Autodesk Inventor part; units mm, degrees
ref_plane "YZ Plane" through (0, 0, 0) normal (1, 0, 0) x (0, 1, 0)
ref_plane "XZ Plane" through (0, 0, 0) normal (0, 1, 0) x (-1, 0, 0)
ref_plane "XY Plane" through (0, 0, 0) normal (0, 0, 1) x (1, 0, 0)
sketch "Szkic1" plane through (0, 0, 0) normal (0, 0, 1) x (1, 0, 0)
  line L0 (-218.2, 284.6) -> (218.2, 284.6)
  line L1 (219.2, 283.6) -> (219.2, 0.3)
  line L2 (218.2, -0.7) -> (-218.2, -0.7)
  line L3 (-219.2, 0.3) -> (-219.2, 283.6)
  arc A0 (219.2, 283.6) -> (218.2, 284.6) centre (218.2, 283.6) ccw
  arc A1 (-218.2, 284.6) -> (-219.2, 283.6) centre (-218.2, 283.6) ccw
  arc A2 (-219.2, 0.3) -> (-218.2, -0.7) centre (-218.2, 0.3) ccw
  arc A3 (218.2, -0.7) -> (219.2, 0.3) centre (218.2, 0.3) ccw
  line L4 (214.5, 280.9) -> (-214.5, 280.9)
  line L5 (-215.5, 279.9) -> (-215.5, 3.3625)
  line L6 (-214.5, 2.3625) -> (214.5, 2.3625)
  line L7 (215.5, 3.3625) -> (215.5, 279.9)
  arc A4 (-214.5, 280.9) -> (-215.5, 279.9) centre (-214.5, 279.9) ccw
  arc A5 (215.5, 279.9) -> (214.5, 280.9) centre (214.5, 279.9) ccw
  arc A6 (214.5, 2.3625) -> (215.5, 3.3625) centre (214.5, 3.3625) ccw
  arc A7 (-215.5, 3.3625) -> (-214.5, 2.3625) centre (-214.5, 3.3625) ccw
  point P0 (0, 0)
  point P1 (219.2, 284.6)
  point P2 (-219.2, -0.7)
  point P3 (219.2, -0.7)
  dimension "d7" = 1
extrude "Wyciągnięcie proste1" add sketch "Szkic1" along normal blind 1.5
sketch "Szkic2" plane through (0, 0, 0) normal (0, 0, -1) x (-1, 0, 0)
  line L0 (217, 2.5) -> (217, 281.4)
  line L1 (216, 282.4) -> (-216, 282.4)
  line L2 (-217, 281.4) -> (-217, 2.5)
  line L3 (-215.5, 3.3625) -> (-215.5, 279.9)
  arc A0 (-214.5, 280.9) -> (-215.5, 279.9) centre (-214.5, 279.9) ccw
  line L4 (-214.5, 280.9) -> (214.5, 280.9)
  arc A1 (215.5, 279.9) -> (214.5, 280.9) centre (214.5, 279.9) ccw
  line L5 (215.5, 279.9) -> (215.5, 3.3625)
  arc A2 (214.5, 2.3625) -> (215.5, 3.3625) centre (214.5, 3.3625) ccw
  line L6 (216, 1.5) -> (73, 1.5)
  line L7 (214.5, 2.3625) -> (-214.5, 2.3625)
  arc A3 (-215.5, 3.3625) -> (-214.5, 2.3625) centre (-214.5, 3.3625) ccw
  line L8 (-51.8, 1.5) -> (-216, 1.5)
  line L9 (-216, 282.4) -> (-215.9969, 282.4)
  line L10 (-39.9, 1.5) -> (-51.8, 1.5)
  line L11 (61.1, 1.5) -> (-39.9, 1.5)
  line L12 (73, 1.5) -> (61.1, 1.5)
  arc A4 (-216, 282.4) -> (-217, 281.4) centre (-216, 281.4) ccw
  arc A5 (217, 281.4) -> (216, 282.4) centre (216, 281.4) ccw
  arc A6 (216, 1.5) -> (217, 2.5) centre (216, 2.5) ccw
  arc A7 (-217, 2.5) -> (-216, 1.5) centre (-216, 2.5) ccw
  point P0 (0, 0)
  dimension "d10" = 1
  dimension "d11" = 1
  dimension "d12" = 1
  dimension "d13" = 1
extrude "Wyciągnięcie proste2" add sketch "Szkic2" along normal blind 5
sketch "Szkic3" plane through (0, 0, 1.5) normal (0, 0, 1) x (1, 0, 0)
  line L0 (-220.2, 284.6) -> (-220.2, -0.7)
  arc A0 (-220.2, -0.7) -> (-219.2, -1.7) centre (-219.2, -0.7) ccw
  line L1 (-219.2, -1.7) -> (219.2, -1.7)
  arc A1 (-219.2, 285.6) -> (-220.2, 284.6) centre (-219.2, 284.6) ccw
  line L2 (219.2, 285.6) -> (-219.2, 285.6)
  arc A2 (220.2, 284.6) -> (219.2, 285.6) centre (219.2, 284.6) ccw
  line L3 (220.2, -0.7) -> (220.2, 284.6)
  arc A3 (219.2, -1.7) -> (220.2, -0.7) centre (219.2, -0.7) ccw
  line L4 (-204.2, 269.6) -> (204.2, 269.6)
  line L5 (204.2, 269.6) -> (204.2, 14.3)
  line L6 (204.2, 14.3) -> (-204.2, 14.3)
  line L7 (-204.2, 14.3) -> (-204.2, 269.6)
  point P0 (0, 0)
extrude "Wyciągnięcie proste4" add sketch "Szkic3" along normal blind 5.2
fillet "Zaokrąglenie2" radius 0.5 8 edges at (-219.9071, 285.3071, 1.5) (-220.2, 141.95, 1.5) (-219.9071, -1.4071, 1.5) (0, -1.7, 1.5) (219.9071, -1.4071, 1.5) (220.2, 141.95, 1.5) (219.9071, 285.3071, 1.5) (0, 285.6, 1.5)
fillet "Zaokrąglenie3" radius 1 8 edges at (-219.9071, 285.3071, 6.7) (-220.2, 141.95, 6.7) (-219.9071, -1.4071, 6.7) (0, -1.7, 6.7) (219.9071, -1.4071, 6.7) (220.2, 141.95, 6.7) (219.9071, 285.3071, 6.7) (0, 285.6, 6.7)
sketch "Szkic4" plane through (0, 0, 1.5) normal (0, 0, -1) x (-1, 0, 0)
  line L0 (-215.5, 3.3625) -> (-215.5, 279.9)
  arc A0 (-214.5, 280.9) -> (-215.5, 279.9) centre (-214.5, 279.9) ccw
  line L1 (-204.2, 14.3) -> (-204.2, 269.6)
  line L2 (-204.2, 269.6) -> (204.2, 269.6)
  line L3 (-214.5, 280.9) -> (214.5, 280.9)
  line L4 (204.2, 269.6) -> (204.2, 14.3)
  arc A1 (215.5, 279.9) -> (214.5, 280.9) centre (214.5, 279.9) ccw
  line L5 (215.5, 279.9) -> (215.5, 3.3625)
  line L6 (204.2, 14.3) -> (-204.2, 14.3)
  line L7 (214.5, 2.3625) -> (-214.5, 2.3625)
  arc A2 (214.5, 2.3625) -> (215.5, 3.3625) centre (214.5, 3.3625) ccw
  arc A3 (-215.5, 3.3625) -> (-214.5, 2.3625) centre (-214.5, 3.3625) ccw
  point P0 (0, 0)
extrude "Wyciągnięcie proste5" add sketch "Szkic4" along normal blind 1.1
chamfer "Faza1" distance 1.5 distance2 1 1 edges at (-204.2, 141.95, 6.7) measured on face at (68.0667, 4.3, 6.7)
chamfer "Faza2" distance 1.5 distance2 1 1 edges at (0, 269.6, 6.7) measured on face at (68.0667, 4.3, 6.7)
chamfer "Faza3" distance 1.5 distance2 1 1 edges at (204.2, 141.95, 6.7) measured on face at (68.0667, 4.3, 6.7)
chamfer "Faza4" distance 1.5 distance2 1 1 edges at (0, 14.3, 6.7) measured on face at (68.0667, 4.3, 6.7)
sketch "Szkic5" plane through (0, 0, 6.7) normal (0, 0, 1) x (1, 0, 0)
  line L0 (219.2, -1.7) -> (206.2, -1.7)
  line L1 (206.2, -1.7) -> (206.45, -1.7)
  line L2 (206.2, 71.425) -> (220.2, 71.425)
  line L3 (220.2, 71.425) -> (220.2, -0.7)
  arc A0 (219.2, -1.7) -> (220.2, -0.7) centre (219.2, -0.7) ccw
  line L4 (206.2, -1.7) -> (206.2, 71.425)
extrude "Wyciągnięcie proste6" cut sketch "Szkic5" against normal blind 6.2
sketch "Szkic6" plane through (0, 0, 6.7) normal (0, 0, 1) x (1, 0, 0)
  line L0 (2.6567, 2.6528) -> (2.657, 4.8393)
  line L1 (-6.8758, 5.3818) -> (-2.1024, 2.2136)
  line L2 (-2.2336, 10.8259) -> (-6.9572, 7.6927)
  line L3 (-2.1024, 2.2136) -> (2.6564, 5.385)
  line L4 (14.4188, 2.6234) -> (14.4191, 4.8375)
  line L5 (1.9087, 8.0765) -> (-1.7626, 5.6414)
  line L6 (1.9087, 8.0765) -> (0.1103, 9.2702)
  line L7 (0.1103, 9.2702) -> (-3.5698, 6.8293)
  line L8 (-3.5698, 6.8293) -> (-4.1314, 7.2021)
  line L9 (-4.1314, 7.2021) -> (-0.4514, 9.643)
  line L10 (-0.4514, 9.643) -> (-2.2336, 10.8259)
  line L11 (14.4188, 2.6234) -> (14.4188, 2.652)
  line L12 (2.6564, 2.6222) -> (2.6564, 5.385)
  line L13 (8.7309, 2.6234) -> (8.7309, 10.6234)
  line L14 (8.7309, 10.6234) -> (11.5831, 10.6234)
  line L15 (8.7309, 10.6234) -> (11.5831, 10.6234)
  line L16 (11.5831, 10.6234) -> (11.5831, 4.8379)
  line L17 (11.5831, 4.8379) -> (14.4191, 4.8375)
  line L18 (14.4188, 2.6234) -> (8.7309, 2.6234)
  line L19 (8.3444, 2.623) -> (2.6564, 2.623)
  line L20 (8.3444, 2.623) -> (8.3447, 4.8375)
  line L21 (5.5087, 4.8379) -> (8.3447, 4.8375)
  line L22 (5.5087, 10.6234) -> (5.5087, 4.8379)
  line L23 (2.6567, 10.6234) -> (5.5087, 10.6234)
  line L24 (2.8855, 10.652) -> (2.5712, 10.652)
  line L25 (2.6564, 2.623) -> (2.6564, 5.385)
  line L26 (2.6567, 7.7426) -> (2.6567, 10.6234)
  line L27 (-14.4194, 2.4022) -> (-14.4194, 10.4022)
  line L28 (-14.4194, 10.4022) -> (-10.5724, 10.4022)
  line L29 (-14.4194, 10.4022) -> (-10.5724, 10.4022)
  line L30 (-14.4194, 2.4022) -> (-10.5724, 2.4022)
  arc A0 (-10.5724, 2.4022) -> (-6.8758, 5.3818) centre (-10.7474, 6.4022) ccw
  arc A1 (-6.9572, 7.6927) -> (-10.5724, 10.4022) centre (-10.7474, 6.4022) ccw
  line L31 (-11.568, 4.7844) -> (-11.568, 7.9195)
  line L32 (-11.568, 7.9195) -> (-10.9818, 7.9195)
  arc A2 (-10.9818, 4.7844) -> (-10.9818, 7.9195) centre (-10.9818, 6.352) ccw
  line L33 (-7.0718, 7.99) -> (-7.0718, 7.9899)
  line L34 (-1.1458, 5.2204) -> (-1.7626, 5.6414)
  line L35 (-1.1458, 5.2204) -> (2.6567, 7.7426)
  line L36 (-11.568, 4.7844) -> (-10.9818, 4.7844)
extrude "Wyciągnięcie proste7" cut sketch "Szkic6" against normal blind 0.01
properties part number "OBUDOWA PRZEDNIA" material "Tworzywo sztuczne, nieprzezroczyste czarne"
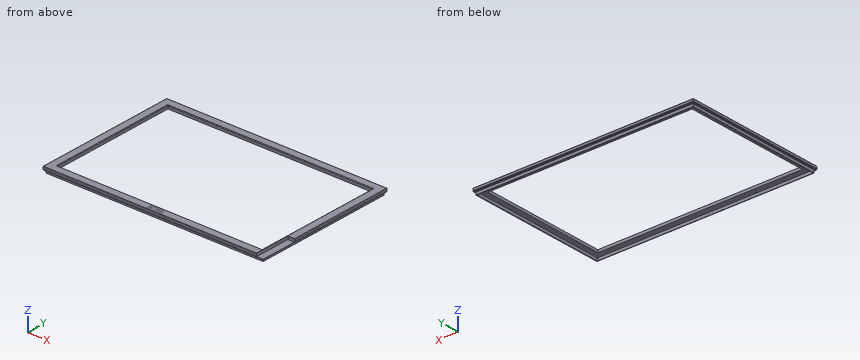
Could you check a few things on this model? Use its own coordinates, in mm. Give positions to 0.01 mm unless a question says otherwise; leave off trailing zeros. Order: outer loops, then holes, each group sorted by start corner. A loop starts at its lowest first (then second) coordinate and runs counter-clockwise, first axis right, second up.
Item 1: If we section it at C-C, the plane y = 172: Write out the boundary of the cut face in (x, z).
Item 2: I'm going to push flat-ended pins straight in: pin 1 (1.5 mm diameter, centred on x = -48, z = 1, fed in from +Y); pin 2 (4 mm diameter, centred on x = 215, y = 48.5, fed in from +Z); pin 3 (3 mm diameter, centred on x = 7.5, z = -3, fed in from +Y). Where does each tip first touch, or does it pass through?
Item 3: If we section it at B-B, the plane z = -2: Write out the boundary of the cut face in (x, y), plus the area to 3 significant figures.
Item 4: I need wall thicknesses on line 1 (Y direction, x = -114.5, z = 3.75); line 2 (Y direction, x = -153, z = 0.75); line 3 (X direction, y = 184, z = -4.25). Which ranges of each line are inside material? Lowest first, please.
Item 5: If we section it at A-A, the plane x = -19: Write out the boundary of the cut face in (y, z), plus the area to 3 significant figures.
Values:
1. outline: (-220.2, 2) arc R0.5 ccw to (-219.7, 1.5) - (-219.2, 1.5) - (-219.2, 0) - (-217, 0) - (-217, -5) - (-215.5, -5) - (-215.5, 0.4) - (-204.2, 0.4) - (-204.2, 5.7) - (-205.7, 6.7) - (-219.2, 6.7) arc R1 ccw to (-220.2, 5.7) - close; (204.2, 0.4) - (215.5, 0.4) - (215.5, -5) - (217, -5) - (217, 0) - (219.2, 0) - (219.2, 1.5) - (219.7, 1.5) arc R0.5 ccw to (220.2, 2) - (220.2, 5.7) arc R1 ccw to (219.2, 6.7) - (205.7, 6.7) - (204.2, 5.7) - close
2. pin 1: stops at y = 285.53
2. pin 2: stops at z = 0.5
2. pin 3: stops at y = 282.4
3. outline: (-217, 2.5) arc R1 ccw to (-216, 1.5) - (216, 1.5) arc R1 ccw to (217, 2.5) - (217, 281.4) arc R1 ccw to (216, 282.4) - (-216, 282.4) arc R1 ccw to (-217, 281.4) - close; hole (-215.5, 3.36) arc R1 ccw to (-214.5, 2.36) - (214.5, 2.36) arc R1 ccw to (215.5, 3.36) - (215.5, 279.9) arc R1 ccw to (214.5, 280.9) - (-214.5, 280.9) arc R1 ccw to (-215.5, 279.9) - close
3. area: 1,860 mm2
4. line 1: y = -1.7 to 14.3, 269.6 to 285.6
4. line 2: y = -0.7 to 14.3, 269.6 to 284.6
4. line 3: x = -217 to -215.5, 215.5 to 217
5. outline: (-1.7, 2) arc R0.5 ccw to (-1.2, 1.5) - (-0.7, 1.5) - (-0.7, 0) - (1.5, 0) - (1.5, -5) - (2.36, -5) - (2.36, 0.4) - (14.3, 0.4) - (14.3, 5.7) - (12.8, 6.7) - (-0.7, 6.7) arc R1 ccw to (-1.7, 5.7) - close; (269.6, 0.4) - (280.9, 0.4) - (280.9, -5) - (282.4, -5) - (282.4, 0) - (284.6, 0) - (284.6, 1.5) - (285.1, 1.5) arc R0.5 ccw to (285.6, 2) - (285.6, 5.7) arc R1 ccw to (284.6, 6.7) - (271.1, 6.7) - (269.6, 5.7) - close
5. area: 212 mm2
